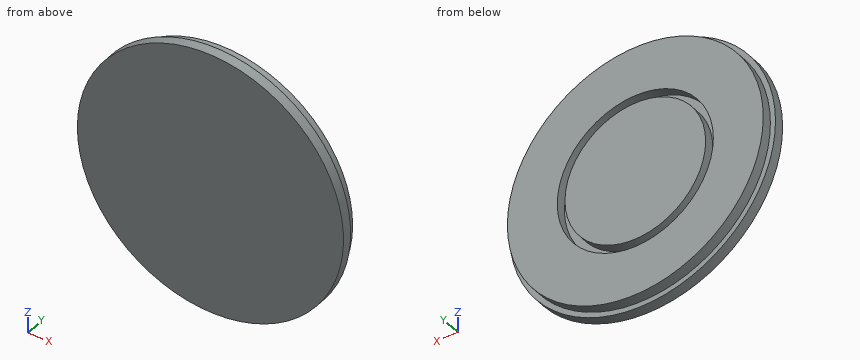
Autodesk Inventor part; units mm, degrees
ref_plane "YZ Plane" through (0, 0, 0) normal (1, 0, 0) x (0, 1, 0)
ref_plane "XZ Plane" through (0, 0, 0) normal (0, 1, 0) x (-1, 0, 0)
ref_plane "XY Plane" through (0, 0, 0) normal (0, 0, 1) x (1, 0, 0)
sketch "Sketch1" plane through (0, 0, 0) normal (0, 1, 0) x (-1, 0, 0)
  circle A0 centre (0, 0) radius 25
  circle A1 centre (0, 0) radius 26
  dimension "d0" = 50
  dimension "d1" = 52
extrude "Extrusion1" add sketch "Sketch1" along normal blind 2 contours A0 | A1
sketch "Sketch2" plane through (0, 2, 0) normal (0, 1, 0) x (1, 0, 0)
  circle A0 centre (0, 0) radius 25
  dimension "d4" = 50
extrude "Extrusion2" add sketch "Sketch2" along normal blind 2
sketch "Sketch3" plane through (0, 4, 0) normal (0, 1, 0) x (1, 0, 0)
  circle A0 centre (0, 0) radius 13.75
  circle A1 centre (0, 0) radius 15.25
  dimension "d7" = 27.5
  dimension "d8" = 30.5
extrude "Extrusion3" cut sketch "Sketch3" against normal blind 2
properties part number "Cap"
For this review, take the finished solid that the model builds, in its own axes (mm). Round coordinates to 2 decimals unless told otherwise and drop trailing zeros. Write each loop counter-clockwise with the first axis right and the second up, starting at its lowest first coordinate (ties: lowest second). Pieces come first, ordered by that corner, then holes. Notation, with made-up numbers: (1, 61.5) -> (11, 61.5) arc R22 cw to (11, 73.5) -> close; hole circle Ø2 at (70, -16). An arc over 180 degrees is marked (long way). Use one line per item in the form item = value.
Q1. Consider section C-C (y = 3.3). State the section outline as (x, z) points.
Resolved:
outline = circle Ø50 at (0, 0); circle Ø27.5 at (0, 0); hole circle Ø30.5 at (0, 0)
Q2. Clearance check with a flat-ended pin moving along its axis: pin 1 Ø1.5 at (y, z) = (0.5, -7) entering from +X. State where the tip first meets the part, or that it passes through.
Resolved:
pin_1 = 25.24
Q3. To check wall thickness, follow probe 1 along Z at (x, y) = (0, 3.05); probe 2 along Z at (x, y) = (-7, 3.3). State the ranges of each line that lie inside material, in increasing order. Write a range as from..to.
Resolved:
probe_1 = -25..-15.25, -13.75..13.75, 15.25..25
probe_2 = -24..-13.55, -11.83..11.83, 13.55..24
Q4. Consider section B-B (z = 0). State the section outline as (x, y) points, then the cut area to 3 significant figures.
Resolved:
outline = (-26, 0) -> (26, 0) -> (26, 2) -> (25, 2) -> (25, 4) -> (15.25, 4) -> (15.25, 2) -> (13.75, 2) -> (13.75, 4) -> (-13.75, 4) -> (-13.75, 2) -> (-15.25, 2) -> (-15.25, 4) -> (-25, 4) -> (-25, 2) -> (-26, 2) -> close
area = 198 mm²
Q5. Consider section A-A (x = 0). State the section outline as (y, z) points, then the cut area to 3 significant figures.
Resolved:
outline = (0, -26) -> (2, -26) -> (2, -25) -> (4, -25) -> (4, -15.25) -> (2, -15.25) -> (2, -13.75) -> (4, -13.75) -> (4, 13.75) -> (2, 13.75) -> (2, 15.25) -> (4, 15.25) -> (4, 25) -> (2, 25) -> (2, 26) -> (0, 26) -> close
area = 198 mm²
